from build123d import *

# Parameters (mm, degrees)
F0_R     = 3.5
F0_R_2   = 2
F1_DEPTH = 10
F2_R     = 3.75
F2_R_2   = 2
F3_DEPTH = 0.5
F4_R     = 5
F4_R_2   = 2
F5_DEPTH = 1
F6_R     = 0.2
F7_SIZE  = 0.7


with BuildPart() as f1:
    # F0 (on Top) → F1 (new body)
    with BuildSketch(Plane.XY):
        Circle(F0_R)
        Circle(F0_R_2, mode=Mode.SUBTRACT)
    extrude(amount=F1_DEPTH)

    # F2 (on face) → F3 (join)
    with BuildSketch(Plane.XY.offset(10)):
        Circle(F2_R)
        Circle(F2_R_2, mode=Mode.SUBTRACT)
    extrude(amount=F3_DEPTH)

    # F4 (on face) → F5 (join)
    with BuildSketch(Plane.XY.offset(10.5)):
        Circle(F4_R)
        Circle(F4_R_2, mode=Mode.SUBTRACT)
    extrude(amount=F5_DEPTH)

    # F6
    f6_edges = [f1.edges().sort_by_distance(p)[0] for p in [
        (-5, 0, 10.5),
        (-5, 0, 11.5),
        (-3.75, 0, 10),
    ]]
    fillet(f6_edges, radius=F6_R)

    # F7
    f7_edges = [f1.edges().sort_by_distance(p)[0] for p in [
        (-3.5, 0, 0),
    ]]
    chamfer(f7_edges, length=F7_SIZE)


solid = f1.part
Read the model definition and answer for the solid it produces. Units are mm, in the model's axes. A direction names the side the tool comes from. Give positions to 0.01 mm unless a question says otherwise; leave off trailing zeros. Write each loop counter-clockwise with the first axis right and the second up, starting at its lowest first coordinate (ties: lowest second). Pieces come first, ordered by that corner, then holes. Notation, with made-up numbers: M 10,-16.5 L 55,-16.5 A12 cw 55,-9.5 Z; hole C -11,7 d10. An arc over 180 degrees is marked long. One line per item, written item: value. Start each with the question number.
(1) Find the intervals of material crossed by line 1 (Y direction, x = 0, z = 2.5); line 2 (X direction, y = 1.25, z = 8.5); line 3 (Z direction, x = 1.5, y = -4), in increasing order.
(2) A tool of negligible diameter and unlimited length cuts with its end or side. For faces 4 (the cylindrical face through (3.233, -1.341, 5.285)), 5 (the flat face through (2, -1, 11.5)), from which of +Z, -Z, +X, -X, +Y, -Y can it reach the whole face along a straight path? Write none if from no direction.
(3) Flat-ended cylindrical pins translate along their axes: pin 1 Ø1 at (y, z) = (0, 6) entering from -X; pin 2 Ø1 at (x, y) = (2, -3) entering from -Z; pin 3 Ø5 at (x, z) = (-3, 7.5) entering from -Y. Find the tip coordinate at first contact, or state that the pin passes through.
(4) Find section D-D (z = 3.75). Determine the outline of the cut face in (x, y).
(5) Find section C-C (z = 11). Determine the outline of the cut face in (x, y).
(6) Determine the mould class of faces 1 (the flat face through (-4, -1, 10.5)), 2 (the cylindrical face through (-1.08, -4.88, 11)), 3 (the cylindrical face through (0, -2, 6)) for opening direction Y: pulls with the +Y half, pulls with the -Y half, needs draft (parallel to the pull), parting line crosses it, or undercut.
(7) Find section A-A (x = 0). Determine the outline of the cut face in (y, z), plus the area to 3 significant figures.
Results below:
1. line 1: y = -3.5 to -2, 2 to 3.5
1. line 2: x = -3.27 to -1.56, 1.56 to 3.27
1. line 3: z = 10.5 to 11.5
2. face 4: -Z
2. face 5: +Z, +X, -X, +Y, -Y
3. pin 1: stops at x = -3.5
3. pin 2: stops at z = 0.31
3. pin 3: stops at y = -3.46
4. outline: C 0,0 d7; hole C 0,0 d4
5. outline: C 0,0 d10; hole C 0,0 d4
6. face 1: needs draft
6. face 2: parting line crosses it
6. face 3: undercut
7. outline: M -5,10.7 A0.2 ccw -4.8,10.5 L -3.75,10.5 L -3.75,10.2 A0.2 ccw -3.55,10 L -3.5,10 L -3.5,0.7 L -2.8,0 L -2,0 L -2,11.5 L -4.8,11.5 A0.2 ccw -5,11.3 Z; M 2,0 L 2.8,0 L 3.5,0.7 L 3.5,10 L 3.55,10 A0.2 ccw 3.75,10.2 L 3.75,10.5 L 4.8,10.5 A0.2 ccw 5,10.7 L 5,11.3 A0.2 ccw 4.8,11.5 L 2,11.5 Z
7. area: 37.2 mm^2
